```python
from build123d import *

# Parameters (mm, degrees)
F1_DEPTH = 6.35
F2_R     = 6.3499
F0_R     = 5.08
F3_DEPTH = 6.35
F4_DEPTH = 6.35


# Not quite as in the source:
# - a fillet or chamfer is up to 0.001 mm smaller than in the source, because OpenCascade refuses the exact size


with BuildPart() as f1:
    # F0 (on Front) → F1 (new body, symmetric)
    with BuildSketch(Plane.XZ):
        with BuildLine():
            Line((12.7, 6.35), (-12.7, 6.35))
            Line((-12.7, 6.35), (-12.7, -6.35))
            Line((-12.7, -6.35), (12.7, -6.35))
            ThreePointArc((12.7, -6.35), (10.471147458, 0), (12.7, 6.35))
        make_face()
        with BuildLine():
            Line((-12.7, -6.35), (-12.7, 6.35))
            ThreePointArc((-12.7, 6.35), (-19.05, 0), (-12.7, -6.35))
        make_face()
    extrude(amount=F1_DEPTH, both=True)

    # F2 (radius 6.35 in the source; OpenCascade refuses exactly that, so slightly less here)
    f2_edges = [f1.edges().sort_by_distance(p)[0] for p in [
        (0, -6.35, 6.35),
        (0, 6.35, 6.35),
        (0, -6.35, -6.35),
        (0, 6.35, -6.35),
    ]]
    fillet(f2_edges, radius=F2_R)

    # F0 (on Front) → F3 (join)
    with BuildSketch(Plane.XZ):
        with BuildLine():
            ThreePointArc((30.791147458, 0), (23.9960502669, 9.5866067556), (12.7, 6.35))
            Line((12.7, 6.35), (12.7, -6.35))
            ThreePointArc((12.7, -6.35), (23.9960502669, -9.5866067556), (30.791147458, 0))
        make_face()
        with Locations((20.631147458, 0)):
            Circle(F0_R, mode=Mode.SUBTRACT)
        with BuildLine():
            Line((12.7, -6.35), (12.7, 6.35))
            ThreePointArc((12.7, 6.35), (10.471147458, 0), (12.7, -6.35))
        make_face()
    extrude(amount=F3_DEPTH)

    # F0 (on Front) → F4 (join, symmetric)
    with BuildSketch(Plane.XZ):
        with Locations((20.631147458, 0)):
            Circle(F0_R)
    extrude(amount=F4_DEPTH, both=True)


solid = f1.part
```
For this review, take the finished solid that the model builds, in its own axes (mm). A direction names the side the tool comes from. Give positions to 0.01 mm unless a question says otherwise; leave off trailing zeros. Order: outer loops, then holes, each group sorted by start corner. A loop starts at its lowest first (then second) coordinate and runs counter-clockwise, first axis right, second up.
1) Take a section at B-B (z = -7.5). Give the boundary of the cut face in (x, y).
2) Insertion check: pin 1 (3 mm diameter, centred on x = -3, z = -7, fed in from -Y); pin 2 (5 mm diameter, centred on x = 4, y = 1, fed in from +Z); pin 3 (8 mm diameter, centred on x = 7, z = 5, fed in from -Y). Each pin has a flat end and moves straight along its axis. Give the tip position at first contact, or say it passes through.
3) For faces 4 (the face through (-0.18, 4.44, 4.54)), 5 (the face through (0.18, -4.44, -4.54)), 6 (the face through (-0.18, -4.44, 4.54)), list the 3-axis set-ups (+Z, -Z, +X, -X, +Y, -Y) from which the entire face can be reached by the end or side of a thin tool; tool diameter is ignored.
4) Take a section at C-C (z = 9). Give the boundary of the cut face in (x, y).
5) The part is to be moulded in two halves that separate along X. For faces 1 (the face through (0.18, 4.44, -4.54)), 2 (the face through (10.47, 2.42, -0.1)), 3 (the face through (23, 0, 5)), say which applies: released by +X, released by -X, zero draft, split by the parting line, or undercut.
6) Wall thickness on line 1 (Y direction, x = 22.5, z = 7.5); line 2 (X direction, y = 4.5, z = -1.75); line 3 (X direction, y = -2, z = -4.75): over which ranges is each line inside the solid? List them lowest first.
Derived:
1. outline: (13.78, -6.35) - (27.49, -6.35) - (27.49, 0) - (13.78, 0) - close
2. pin 1: stops at y = -3.17
2. pin 2: stops at z = 6.35
2. pin 3: stops at y = -6.27
3. face 4: +Z, -X, +Y
3. face 5: -Z, -X, -Y
3. face 6: +Z, -X, -Y
4. outline: (15.92, -6.35) - (25.35, -6.35) - (25.35, 0) - (15.92, 0) - close
5. face 1: zero draft
5. face 2: undercut
5. face 3: undercut
6. line 1: y = -6.35 to 0
6. line 2: x = -16.82 to 10.62, 15.86 to 25.4
6. line 3: x = -16.41 to 29.61
